Could you check a few things on this model? Use its own coordinates, in mm. Round coordinates to 2 decimals unless told otherwise and drop trailing zeros. Write each loop counter-clockwise with the first axis right and the second up, starting at its lowest first coordinate (ties: lowest second). Pieces come first, ordered by that corner, then holes. Notation, with made-up numbers: (-10.75, 78.25) -> (46.25, 78.25) arc R24 ccw to (46.25, 102.25) -> close; hole circle Ø5 at (-33.75, -5.5). An arc over 180 degrees is marked (long way). Answer as CSV lines item,"result". Start each with the question number.
Q1. Imagine slicing it at B-B on z = 0. Please give me the cut outline in (x, y), and give its area (3 significant figures).
Q2. Imagine slicing it at A-A on x = 0. Please give me the cut outline in (y, z).
Q3. Imagine slicing it at C-C on y = 2.6. Give the number of separate pieces and of enclosed holes in the cut face, and give its area (3 significant figures).
Q4. If we mould it in two halves opening along Z, with no side actions, what happens to faces 1 (the flat face through (-11, 0, -38)), 2 (the cylindrical face through (-44.83, 1.01, 14.12)), 3 (the cylindrical face through (29.43, 1.97, 31.78))? For each: pulls with the +Z half, pulls with the -Z half, needs draft (parallel to the pull), parting line crosses it, or undercut.
Q5. Will these pins go through, and if not, where does the flat tip stop? pin 1 Ø2 at (y, z) = (1.5, -26.5) entering from -X; pin 2 Ø1.5 at (y, z) = (3.5, -24.5) entering from -X; pin 3 Ø6.5 at (x, z) = (-42, 0) entering from -Y; pin 4 Ø2 at (x, z) = (35, 30.5) entering from +Y.
Q6. If I drill on line 1 (Z direction, x = 0, y = 1.25); line 2 (X direction, y = 0.65, z = -30.5); line 3 (Z direction, x = 30.5, y = 2.9), over which ranges is the centre line in solid material (lowest first)? Write a range as [from, to].
from build123d import *

# Parameters (mm, degrees)
SKETCH_2_R          = 2.1
CUT_EXTRUDE_1_DEPTH = 10


with BuildPart() as part:
    # 草图1 → 旋转1 (revolve)
    with BuildSketch(Plane.XY):
        Polygon((-39, 0), (-47, 0), (-47, 2), (-45, 4), (-39, 4), align=None)
    revolve(axis=Axis((0, 0, 0), (0, 1, 0)))

    # 草图2 → 切除-拉伸1 (cut)
    with BuildSketch(Plane.XZ):
        with Locations((0, 42)):
            Circle(SKETCH_2_R)
        with Locations((29.69848481, 29.69848481)):
            Circle(SKETCH_2_R)
        with Locations((42, 0)):
            Circle(SKETCH_2_R)
        with Locations((29.69848481, -29.69848481)):
            Circle(SKETCH_2_R)
        with Locations((0, -42)):
            Circle(SKETCH_2_R)
        with Locations((-29.69848481, -29.69848481)):
            Circle(SKETCH_2_R)
        with Locations((-42, 0)):
            Circle(SKETCH_2_R)
        with Locations((-29.69848481, 29.69848481)):
            Circle(SKETCH_2_R)
    extrude(amount=-CUT_EXTRUDE_1_DEPTH, mode=Mode.SUBTRACT)


solid = part.part
Checks:
1,outline,"(-47, 0) -> (-44.1, 0) -> (-44.1, 4) -> (-45, 4) -> (-47, 2) -> close; (-39.9, 0) -> (-39, 0) -> (-39, 4) -> (-39.9, 4) -> close; (39, 0) -> (39.9, 0) -> (39.9, 4) -> (39, 4) -> close; (44.1, 0) -> (47, 0) -> (47, 2) -> (45, 4) -> (44.1, 4) -> close"
1,area,"26.4 mm^2"
2,outline,"(0, -47) -> (2, -47) -> (4, -45) -> (4, -44.1) -> (0, -44.1) -> close; (0, -39.9) -> (4, -39.9) -> (4, -39) -> (0, -39) -> close; (0, 39) -> (4, 39) -> (4, 39.9) -> (0, 39.9) -> close; (0, 44.1) -> (4, 44.1) -> (4, 45) -> (2, 47) -> (0, 47) -> close"
3,separate pieces,"1"
3,enclosed holes,"9"
3,area,"1,870 mm^2"
4,face 1,"needs draft"
4,face 2,"parting line crosses it"
4,face 3,"undercut"
5,pin 1,"x = -39.48"
5,pin 2,"x = -39.34"
5,pin 3,"y = 0"
5,pin 4,"y = 3.58"
6,line 1,"[-47, -44.1], [-39.9, -39], [39, 39.9], [44.1, 47]"
6,line 2,"[-35.76, -31.64], [-27.76, -24.31], [24.31, 27.76], [31.64, 35.76]"
6,line 3,"[-34.57, -31.64], [-27.76, -24.31], [24.31, 27.76], [31.64, 34.57]"
